```python
from build123d import *

# Parameters (mm, degrees)
F3_W         = 38.5
F3_H         = 34
F3_W_2       = 8.5
F3_H_2       = 4
F4_DEPTH     = 15.501
F5_T4_ANGLE  = 146.9201983829
F5_S5_R      = 2.45
F5_T6_DEPTH  = 4
F5_T10_ANGLE = 146.9201983829
F5_S11_R     = 2.45
F5_T12_DEPTH = 4
F5_T14_ANGLE = 146.9201983829
F5_T16_ANGLE = 146.9201983829
F6_W         = 6
F6_H         = 1.4
F7_DEPTH     = 4.001


# Not quite as in the source:
# - a fillet or chamfer that OpenCascade refuses, or shapes differently, is made with other operations: its cross-section is extruded or revolved along the edge and cut away or added


with BuildPart() as f2:
    # F1 (on Front) → F2 (revolve)
    with BuildSketch(Plane.XZ):
        Polygon((0, 7.5), (0, 0), (15.5, 0), (15.5, 2.75), (14.2, 2.75), (14.2, 2.45), (2.2, 2.45), (2.2, 7.5), align=None)
    revolve(axis=Axis((8.8834212145, 0, 0), (1, 0, 0)))

    # F3 (on Right) → F4 (cut, through all)
    with BuildSketch(Plane.YZ):
        Rectangle(F3_W, F3_H)
        Rectangle(F3_W_2, F3_H_2, mode=Mode.SUBTRACT)
    extrude(amount=F4_DEPTH, mode=Mode.SUBTRACT)

    # F5: chamfer of 0.5 on 4 edges, made by hand


with BuildPart() as f5_tool2:
    # F5_s3 → F5_t4 (revolve)
    with BuildSketch(Plane(origin=(0, 0, 0), x_dir=(1, 0, 0), z_dir=(0, -0.958621714, -0.2846829983))):
        Polygon((14.2, -2.25), (14.7, -2.75), (14.2, -2.75), align=None)
    revolve(axis=Axis((14.2, 0, 0), (1, 0, 0)), revolution_arc=F5_T4_ANGLE)

    # F5_s5 → F5_t6 (cut, symmetric)
    with BuildSketch(Plane.YZ.offset(14.4)):
        Circle(F5_S5_R)
    extrude(amount=F5_T6_DEPTH, both=True, mode=Mode.SUBTRACT)


with BuildPart() as f2_1:
    add(f2.part)

    # F5_t1: cut F5_tool2
    add(f5_tool2.part, mode=Mode.SUBTRACT)


with BuildPart() as f5_tool8:
    # F5_s9 → F5_t10 (revolve)
    with BuildSketch(Plane(origin=(0, 0, 0), x_dir=(1, 0, 0), z_dir=(0, 0.958621714, 0.2846829983))):
        Polygon((14.7, -2.75), (14.2, -2.25), (14.2, -2.75), align=None)
    revolve(axis=Axis((14.2, 0, 0), (1, 0, 0)), revolution_arc=F5_T10_ANGLE)

    # F5_s11 → F5_t12 (cut, symmetric)
    with BuildSketch(Plane.YZ.offset(14.4)):
        Circle(F5_S11_R)
    extrude(amount=F5_T12_DEPTH, both=True, mode=Mode.SUBTRACT)


with BuildPart() as f2_2:
    add(f2_1.part)

    # F5_t7: cut F5_tool8
    add(f5_tool8.part, mode=Mode.SUBTRACT)

    # F5_s13 → F5_t14 (revolve, cut)
    with BuildSketch(Plane(origin=(0, 0, 0), x_dir=(1, 0, 0), z_dir=(0, -0.958621714, -0.2846829983))):
        Polygon((15, -2.75), (15.5, -2.25), (15.5, -2.75), align=None)
    revolve(axis=Axis((15.5, 0, 0), (1, 0, 0)), revolution_arc=F5_T14_ANGLE, mode=Mode.SUBTRACT)

    # F5_s15 → F5_t16 (revolve, cut)
    with BuildSketch(Plane(origin=(0, 0, 0), x_dir=(1, 0, 0), z_dir=(0, 0.958621714, 0.2846829983))):
        Polygon((15.5, -2.25), (15, -2.75), (15.5, -2.75), align=None)
    revolve(axis=Axis((15.5, 0, 0), (1, 0, 0)), revolution_arc=F5_T16_ANGLE, mode=Mode.SUBTRACT)

    # F6 (on face) → F7 (cut, through all)
    with BuildSketch(Plane.XY.offset(2)):
        with Locations((12.5, 0)):
            Rectangle(F6_W, F6_H)
    extrude(amount=-F7_DEPTH, mode=Mode.SUBTRACT)


solid = f2_2.part
```
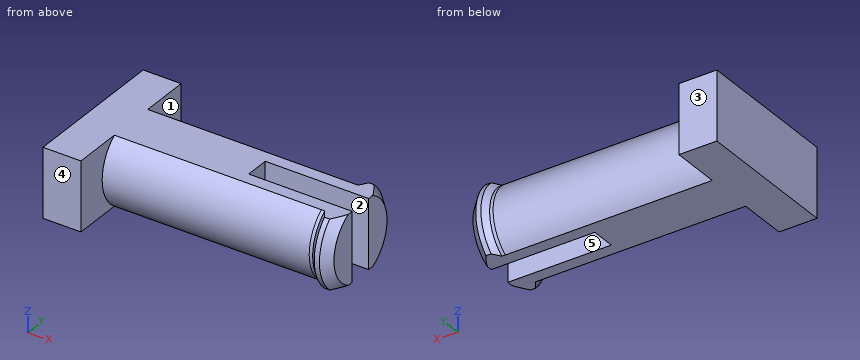
The model under review builds one solid part; all positions refer to its coordinate system, in mm. Face numbers are marked on the shaded views. A direction names the side the tool comes from. Round coordinates to 2 decimals unless told otherwise and drop trailing zeros. Loops run counter-clockwise (first coordinate to the right, second up) from the corner with the lowest first, then second, coordinate; pieces in that order, holes last. Notation, with made-up numbers: M -1.75,7 L 48.25,7 A28 cw 48.25,34 Z; hole C 33,77 d6. An arc over 180 degrees is marked long. Answer as a JSON object with one key per item and string values.
(1) Clearance check with flat-ended pins moving along their axes: P1, Ø1.5, axis at x = 3.5, z = -1.5, coming from the -Y side; P2, Ø2, axis at x = 14, z = -1, coming from the +Y side; P3, Ø1, axis at x = 5, z = 1, coming from the +Y side. State where each tip first meets the part, or that it passes through.
Resolved:
{"P1": "y = -2.33", "P2": "y = 2.74", "P3": "y = 2.4"}
(2) Draft analysis for pull direction Y (two halves, no side actions). For the marked faces 1, 2 and 3, state which applies: released by +Y, released by -Y, zero draft, split by the parting line, or undercut.
Resolved:
{"face 1": "zero draft", "face 2": "undercut", "face 3": "released by +Y"}
(3) Take a section at C-C on x = 5. Give the boundary of the cut face in (y, z).
Resolved:
{"outline": "M -1.42,-2 L 1.42,-2 A2.45 ccw 1.42,2 L -1.42,2 A2.45 ccw Z"}
(4) To check wall thickness, follow line 1 along Y through (x, z) = (11.5, 1.6); line 2 along X through (y, z) = (4, -1.7); line 3 along Y through (x, z) = (14.25, -1.45). State the ranges of each line that lie inside material, in increasing order.
Resolved:
{"line 1": "-1.86 to -0.7, 0.7 to 1.86", "line 2": "0 to 2.2", "line 3": "-1.97 to -0.7, 0.7 to 1.97"}
(5) Take a section at B-B on y = 3.75. Give the boundary of the cut face in (x, z), and give its area (3 significant figures).
Resolved:
{"outline": "M 0,-2 L 2.2,-2 L 2.2,2 L 0,2 Z", "area": "8.80 mm²"}
(6) Take a section at A-A on x = 13.5. Give the boundary of the cut face in (y, z).
Resolved:
{"outline": "M -1.42,-2 L -0.7,-2 L -0.7,2 L -1.42,2 A2.45 ccw Z; M 0.7,-2 L 1.42,-2 A2.45 ccw 1.42,2 L 0.7,2 Z"}
(7) Tool access review of the marked faces 4 and 5: name each direction out of +Z, -Z, +X, -X, +Y, -Y from which nothing blocks a thin tool from reaching the whole face with its end or side.
Resolved:
{"face 4": "+Z, -Z, +X, -X, -Y", "face 5": "+Z, -Z, +X"}
